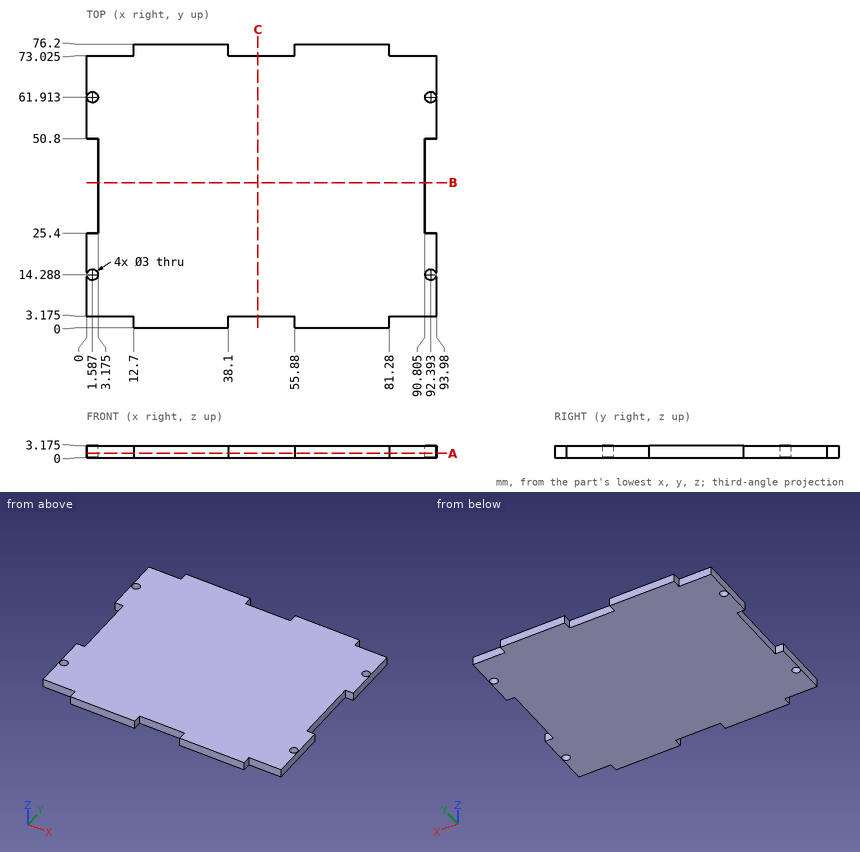
Could you check a few things on this drawing? It's one solid part, dimensions in mm from its lowest x, y, z. Give positions to 0.01 mm unless a question says otherwise; leave off trailing zeros. Write each loop counter-clockwise with the first axis right and the second up, starting at its lowest first coordinate (ties: lowest second). Pieces come first, ordered by that corner, then holes.
(1) If I drill on L1, parallel to X at y = 41, z = 0.8 (1 decimal); L2, parallel to Y at x = 53.5, z = 3 (1 decimal), over which ranges is the centre line in solid material (lowest first)?
Output values:
L1: x = 3.2 to 90.8
L2: y = 3.2 to 73
(2) Imagine slicing it at B-B, the plane y = 39. Write out the boundary of the cut face in (x, z) (1 decimal), and give its area (3 significant figures).
Output values:
outline: (3.2, 0) - (90.8, 0) - (90.8, 3.2) - (3.2, 3.2) - close
area: 278 mm2
(3) Imagine slicing it at C-C, the plane x = 46. Write out the boundary of the cut face in (y, z) (1 decimal).
Output values:
outline: (3.2, 0) - (73, 0) - (73, 3.2) - (3.2, 3.2) - close
(4) Imagine slicing it at A-A, the plane z = 1.15. Count the separate pieces of the cut face and the enclosed holes in it, and give its area (3 significant figures).
Output values:
separate pieces: 1
enclosed holes: 4
area: 6,700 mm2
(5) Will these pins go through, and if not, where does the flat tip stop? pin 1 (1 mm diameter, centred on y = 32, z = 2, fed in from -X) (1 decimal); pin 2 (1.6 mm diameter, centred on y = 1.5, z = 1.5, fed in from +X); pin 3 (1.6 mm diameter, centred on x = 9, z = 2, fed in from +Y) (1 decimal).
Output values:
pin 1: stops at x = 3.2
pin 2: stops at x = 81.28
pin 3: stops at y = 73
